Verification items for the finished model (mm, model axes). Round coordinates to 2 decimals unless told otherwise and drop trailing zeros. Order: outer loops, then holes, each group sorted by start corner. A loop starts at its lowest first (then second) coordinate and runs counter-clockwise, first axis right, second up. Notation, with made-up numbers: M 89,21.25 L 105,21.25 A28 ccw 105,51.25 Z; hole C 2.25,0 d10. An arc over 180 degrees is marked long. One line per item, written item: value. Start each with the question number.
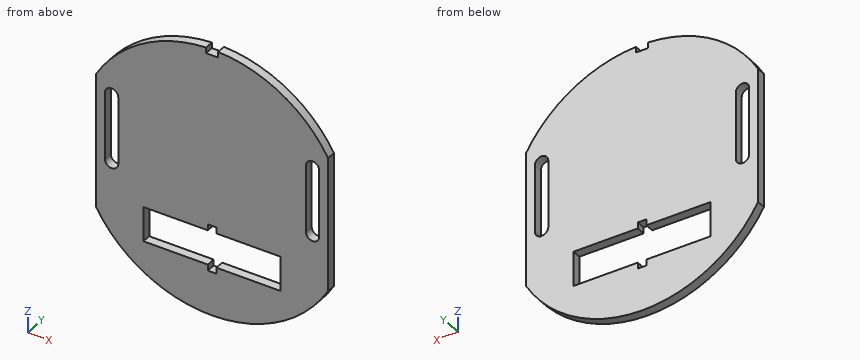
from build123d import *

# Parameters (mm, degrees)
BASE_DEPTH                 = 2.7
WHEEL_HOLE_REACH           = 54.984
BATTERY_HOLE_REACH         = 54.984
IR_SENSOR_DIVOT_DEPTH      = 53.983865469
IR_SENSOR_DIVOT_DEPTH_BACK = 53.983865469


with BuildPart() as part:
    # Sketch1 → Base (new body)
    with BuildSketch(Plane(origin=(0, 0, 0), x_dir=(1, 0, 0), z_dir=(0, 1, 0))):
        with BuildLine():
            Line((34.641016151, 20), (34.641016151, -20))
            ThreePointArc((34.641016151, -20), (0, -40), (-34.641016151, -20))
            Line((-34.641016151, -20), (-34.641016151, 20))
            ThreePointArc((-34.641016151, 20), (0, 40), (34.641016151, 20))
        make_face()
    extrude(amount=BASE_DEPTH)

    # Sketch2 → Wheel Hole (cut, up to next)
    with BuildSketch(Plane(origin=(0, 2.7, 0), x_dir=(-1, 0, 0), z_dir=(0, 1, 0)), mode=Mode.PRIVATE) as wheel_hole_sk1:
        with BuildLine():
            Line((28, -4.65), (28, 15.35))
            ThreePointArc((28, 15.35), (30, 17.35), (32, 15.35))
            Line((32, 15.35), (32, -4.65))
            ThreePointArc((32, -4.65), (30, -6.65), (28, -4.65))
        make_face()
    wheel_hole_tool1 = extrude(wheel_hole_sk1.sketch, amount=-WHEEL_HOLE_REACH, mode=Mode.PRIVATE) & part.part
    wheel_hole = wheel_hole_tool1.solids().sort_by_distance((-30, 2.7, 5.35))[0]
    add(wheel_hole, mode=Mode.SUBTRACT)

    # Sketch6 → Battery Hole (cut, up to next)
    with BuildSketch(Plane(origin=(0, 2.7, 0), x_dir=(-1, 0, 0), z_dir=(0, 1, 0)), mode=Mode.PRIVATE) as battery_hole_sk1:
        Polygon((1.27, -14.85), (1.27, -13.05), (-1.27, -13.05), (-1.27, -14.85), (-20.5, -14.85), (-20.5, -25.15), (-1.27, -25.15), (-1.27, -26.95), (1.27, -26.95), (1.27, -25.15), (20.5, -25.15), (20.5, -14.85), align=None)
    battery_hole_tool1 = extrude(battery_hole_sk1.sketch, amount=-BATTERY_HOLE_REACH, mode=Mode.PRIVATE) & part.part
    add(battery_hole_tool1.solids().sort_by_distance((0, 2.7, -20))[0], mode=Mode.SUBTRACT)

    # Mirror 2: Wheel Hole across plane
    add(wheel_hole.mirror(Plane(origin=(0, 0, 0), x_dir=(0, 0, 1), z_dir=(1, 0, 0))), mode=Mode.SUBTRACT)

    # Sketch5 → IR Sensor Divot (cut, two sides: drawn at the far end of the back side and taken through both)
    with BuildSketch(Plane(origin=(0, 2.7, 0), x_dir=(-1, 0, 0), z_dir=(0, 1, 0)).offset(-IR_SENSOR_DIVOT_DEPTH_BACK)):
        Polygon((-1.8, 225.703224926), (-1.8, 39.959479476), (-1.8, 38.259479476), (1.8, 38.259479476), (1.8, 39.959479476), (1.8, 225.703224926), (1.8, 597.190715827), (-1.8, 597.190715827), align=None)
    extrude(amount=IR_SENSOR_DIVOT_DEPTH + IR_SENSOR_DIVOT_DEPTH_BACK, mode=Mode.SUBTRACT)


solid = part.part
1. Section check D-D (z = -33.5). Record the cut outline in (x, y).
2. Depth check by flat-ended pin: pin 1 (1.4 mm diameter, centred on y = 1.5, z = -26, fed in from +X); pin 2 (0.5 mm diameter, centred on y = 1, z = -26.5, fed in from -X); pin 3 (5 mm diameter, centred on x = 23, z = 30, fed in from -Y); pin 4 (0.8 mm diameter, centred on x = 11, y = 1, fed in from +Z). Enter the tip coordinate at first touch or a pass-through.
3. Scan lines: line 1 along X through (y, z) = (0.95, 1); line 2 along X through (y, z) = (2.2, -6); line 3 along Z through (x, y) = (2, 0.55). Record each from-to range of solid material in increasing order.
4. Section check C-C (x = -5.5). Record the cut outline in (y, z).
5. Section check A-A (y = 1.6). Record the cut outline in (x, z).
6. Section check B-B (z = -16). Record the cut outline in (x, y), and give its area (3 significant figures).
Geometry check:
1. outline: M -21.86,0 L 21.86,0 L 21.86,2.7 L -21.86,2.7 Z
2. pin 1: stops at x = 30.98
2. pin 2: stops at x = -30.18
2. pin 3: stops at y = 0
2. pin 4: stops at z = 38.57
3. line 1: x = -34.64 to -32, -28 to 28, 32 to 34.64
3. line 2: x = -34.64 to -31.48, -28.52 to 28.52, 31.48 to 34.64
3. line 3: z = -39.95 to -25.15, -14.85 to 39.95
4. outline: M 0,-39.62 L 2.7,-39.62 L 2.7,-25.15 L 0,-25.15 Z; M 0,-14.85 L 2.7,-14.85 L 2.7,39.62 L 0,39.62 Z
5. outline: M -34.64,-20 A40 ccw 34.64,-20 L 34.64,20 A40 ccw 1.8,39.96 L 1.8,38.26 L -1.8,38.26 L -1.8,39.96 A40 ccw -34.64,20 Z; hole M -32,-4.65 A2 ccw -28,-4.65 L -28,15.35 A2 ccw -32,15.35 Z; hole M -20.5,-25.15 L -1.27,-25.15 L -1.27,-26.95 L 1.27,-26.95 L 1.27,-25.15 L 20.5,-25.15 L 20.5,-14.85 L 1.27,-14.85 L 1.27,-13.05 L -1.27,-13.05 L -1.27,-14.85 L -20.5,-14.85 Z; hole M 28,-4.65 A2 ccw 32,-4.65 L 32,15.35 A2 ccw 28,15.35 Z
6. outline: M -34.64,0 L -20.5,0 L -20.5,2.7 L -34.64,2.7 Z; M 20.5,0 L 34.64,0 L 34.64,2.7 L 20.5,2.7 Z
6. area: 76.4 mm²
